Autodesk Inventor part; units mm, degrees
ref_plane "YZ Plane" through (0, 0, 0) normal (1, 0, 0) x (0, 1, 0)
ref_plane "XZ Plane" through (0, 0, 0) normal (0, 1, 0) x (-1, 0, 0)
ref_plane "XY Plane" through (0, 0, 0) normal (0, 0, 1) x (1, 0, 0)
sketch "Sketch1" plane through (0, 0, 0) normal (0, 1, 0) x (-1, 0, 0)
  line L0 (0, 0) -> (72.0519, -110.6962) construction
  line L1 (0, 0) -> (0, -132.08) construction
  arc A0 (-1.4091, -0.9301) -> (-42.2635, -176.856) centre (72.0519, -110.6962) ccw
  line L2 (72.0519, -110.6962) -> (-42.2635, -176.856) construction
  arc A1 (0, 22.1526) -> (-15.8725, 12.2248) centre (72.0519, -110.6962) ccw construction
  line L3 (0, 0) -> (-15.9623, 24.5235) construction
  line L4 (0, 1.7085) -> (0, 117.475)
  line L5 (-15.8725, 13.8467) -> (-15.8725, 117.475)
  line L6 (-3.175, 120.65) -> (-12.6975, 120.65)
  line L7 (-49.4275, -181.0021) -> (-64.4319, -173.8454)
  arc A2 (-17.173, 11.2841) -> (-65.9645, -172.2733) centre (72.0519, -110.6962) ccw
  line L8 (-42.2635, -176.856) -> (-41.282, -178.374)
  line L9 (-45.3151, -182.9636) -> (-49.4275, -181.0021)
  arc A3 (-45.3151, -182.9636) -> (-41.282, -178.374) centre (-43.9482, -180.0979) ccw
  arc A4 (-65.9645, -172.2733) -> (-64.4319, -173.8454) centre (-63.065, -170.9797) ccw
  arc A5 (-1.4091, -0.9301) -> (0, 1.7085) centre (-3.175, 1.7085) ccw
  arc A6 (-17.173, 11.2841) -> (-15.8725, 13.8467) centre (-19.0475, 13.8467) ccw
  arc A7 (0, 117.475) -> (-3.175, 120.65) centre (-3.175, 117.475) ccw
  arc A8 (-12.6975, 120.65) -> (-15.8725, 117.475) centre (-12.6975, 117.475) ccw
  point P0 (-65.4815, -173.3448)
  point P1 (0, 120.65)
  point P2 (-35.1928, -187.7917)
  dimension "d1" = 132.08
  dimension "d2" = 33.06
  dimension "d3" = 87
  dimension "d4" = 302.26
  dimension "d5" = 29.2608
  dimension "d6" = 120.65
  dimension "d8" = 3.175
  dimension "d9" = 3.175
  dimension "d10" = 3.175
extrude "Extrusion1" add sketch "Sketch1" along normal blind 3.175
sketch "Sketch2" plane through (0, 3.175, 0) normal (0, 1, 0) x (1, 0, 0)
  arc A0 (17.173, -11.2841) -> (65.9645, 172.2733) centre (-72.0519, 110.6962) ccw
  line L0 (45.6255, 15.8684) -> (-72.0519, 110.6962)
  circle A1 centre (-72.0519, 110.6962) radius 151.13
  circle A2 centre (-72.0519, 110.6962) radius 132.0211
  circle A3 centre (-72.0519, 110.6962) radius 141.605
  circle A4 centre (57.9094, 166.9283) radius 3.175
  arc A5 (17.173, -11.2841) -> (15.8725, -13.8467) centre (19.0475, -13.8467) ccw
  line L1 (0, 0) -> (19.0475, -13.8467)
  circle A6 centre (8.2082, -5.967) radius 3.175
  line L2 (3.175, -120.65) -> (12.6975, -120.65)
  line L3 (7.9363, -120.65) -> (7.9363, 5.6655)
  circle A7 centre (7.9363, -107.95) radius 3.175
  dimension "d13" = 283.21
  dimension "d14" = 6.35
  dimension "d15" = 6.35
  dimension "d16" = 6.35
  dimension "d17" = 12.7
hole "Hole1" at (7.9363, 3.175, 107.95) at (8.2082, 3.175, 5.967) at (57.9094, 3.175, -166.9283) direction (0, -1, 0) diameter 6.35 depth 25.4 tip angle 118
properties part number "2AM-17-P-5201 - claw arm" material "Aluminum 6061"
Verification items for the finished model (mm, model axes). Coordinates: 2 decimals unless noted, no trailing zeros. Order: outer loops, then holes, each group sorted by start corner. A loop starts at its lowest first (then second) coordinate and runs counter-clockwise, first axis right, second up. Notation, with made-up numbers: M 75.5,18.5 L 131.5,18.5 A4 ccw 131.5,22.5 Z; hole C 39.25,12 d11. An arc over 180 degrees is marked long. Write each question's results on one line, items separated by ' | '.
1) Section check B-B on y = 2.55. Give the number of separate pieces and of enclosed holes in the cut face, plus the area to 3 significant figures.
Solved:
separate pieces: 1 | enclosed holes: 3 | area: 5,700 mm²
2) Scan lines: line 1 along X through (y, z) = (1.3, 107.95); line 2 along X through (y, z) = (0.95, 25); line 3 along X through (y, z) = (2.9, -167.5). Record each from-to range of solid material in increasing order. Write a range as [from, to].
Solved:
line 1: x = [0, 4.76], [11.11, 15.87] | line 2: x = [0, 15.87] | line 3: x = [47.19, 54.79], [61.03, 68]
3) Release check for a two-part mould opening along Z. For faces 1 (the face through (57.8, 1.6, -170.1)), 2 (the face through (74.37, 1.57, -73.26)), 3 (the face through (49, 3.175, -42)) record: pulls with the +Z half, pulls with the -Z half, needs draft (parallel to the pull), parting line crosses it, or undercut.
Solved:
face 1: undercut | face 2: parting line crosses it | face 3: needs draft
4) Section check C-C on z = 31.5. Record the cut outline in (x, y) (1 decimal), plus the area to 3 significant figures.
Solved:
outline: M 0,0 L 15.9,0 L 15.9,3.2 L 0,3.2 Z | area: 50.4 mm²
5) Section check A-A on z = 107.95. Record the cut outline in (x, y) (1 decimal), plus the area to 3 significant figures.
Solved:
outline: M 0,0 L 4.8,0 L 4.8,3.2 L 0,3.2 Z; M 11.1,0 L 15.9,0 L 15.9,3.2 L 11.1,3.2 Z | area: 30.2 mm²
6) Section check D-D on x = 71. Record the cut outline in (y, z) (3 decimals).
Solved:
outline: M 0,-159.445 L 3.175,-159.445 L 3.175,-61.948 L 0,-61.948 Z
7) Gauge pin test, flat ends, axial feed: pin 1 Ø1.5 at (y, z) = (1.5, -87) entering from +X; pin 2 Ø10 at (x, z) = (7.94, 107.95) entering from +Y (3 decimals); pin 3 Ø1 at (x, y) = (53, 1.5) entering from +Z. Record the tip position at first contact, or that the pin passes through.
Solved:
pin 1: stops at x = 77.33 | pin 2: stops at y = 3.175 | pin 3: stops at z = -25.1
